from build123d import *

# Parameters (mm, degrees)
SKETCH_W        = 95
SKETCH_H        = 900
PAD_DEPTH       = 45
SKETCH001_W     = 95
SKETCH001_H     = 95
SKETCH001_W_2   = 22.5
SKETCH001_H_2   = 47.5
POCKET_DEPTH    = 22.5
SKETCH011_W     = 22.5
SKETCH011_H     = 47.5
POCKET006_DEPTH = 22.5


with BuildPart() as part:
    # Sketch → Pad (new body)
    with BuildSketch(Plane.XY):
        with Locations((47.5, 450)):
            Rectangle(SKETCH_W, SKETCH_H)
    extrude(amount=-PAD_DEPTH)

    # Sketch001 (on Face5 of Pad) → Pocket (cut)
    with BuildSketch(Plane.XY):
        with Locations((47.5, 167.5)):
            Rectangle(SKETCH001_W, SKETCH001_H)
        with Locations((47.5, 852.5)):
            Rectangle(SKETCH001_W, SKETCH001_H)
        with Locations((47.5, 333.75)):
            Rectangle(SKETCH001_W_2, SKETCH001_H_2)
    extrude(amount=-POCKET_DEPTH, mode=Mode.SUBTRACT)

    # Sketch011 (on Face4 of Pocket) → Pocket006 (cut)
    with BuildSketch(Plane(origin=(0, 0, -45), x_dir=(1, 0, 0), z_dir=(0, 0, -1))):
        with Locations((47.5, -333.75)):
            Rectangle(SKETCH011_W, SKETCH011_H)
    extrude(amount=-POCKET006_DEPTH, mode=Mode.SUBTRACT)


solid = part.part
Input: part model. Units: mm. Frame: model coordinates. A direction names the side the tool comes from. Round coordinates to 2 decimals unless told otherwise and drop trailing zeros. Order: outer loops, then holes, each group sorted by start corner. A loop starts at its lowest first (then second) coordinate and runs counter-clockwise, first axis right, second up. Notation, with made-up numbers: (22, 88) - (30, 88) arc R6 cw to (30, 94) - close; hole circle Ø5 at (-23, 1). An arc over 180 degrees is marked (long way). Answer as a JSON object with one key per item and string values. Group by question number.
(1) Cut plane D-D (y = 130.5). Return loops of the section in (x, z), then the cut area to 3 significant figures.
(2) Reachability of faces 1 (the face through (47, 310, -22)), 2 (the face through (47, 853, -22.5)), 3 (the face through (47, 215, -11)), 4 (the face through (47, 61, 0)) from +Z, -Z, +X, -X, +Y, -Y: full face, straight path, thin tool, end or side. Return the list, or none.
(3) Draft query along Y for faces 5 (the face through (47, 120, -11)), 6 (the face through (47, 805, -11)), 7 (the face through (47, 456, -45)). Return one class per face: released by +Y, released by -Y, zero draft, split by the parting line, or undercut.
(4) Cut plane A-A (z = -14). Return loops of the section in (x, y).
(5) Material intervals for probe 1 along Y at (x, z) = (76, -19.5); probe 2 along Y at (x, z) = (47, -18); probe 3 along Y at (x, z) = (42.5, -42.5), sorted ascending. Write a range as from..to.
(6) Cut plane B-B (x = 72). Return loops of the section in (y, z), then the cut area to 3 significant figures.
(7) Cut plane C-C (y = 318.5). Return loops of the section in (x, z).
(8) Pin query (flat end, axial travel): P1, Ø18, axis at x = 50, z = -12, coming from the +Y side. Return the tip coordinate at first contact, or that it passes through.
Here are the results:
{
 "1": {"outline": "(0, -45) - (95, -45) - (95, -22.5) - (0, -22.5) - close", "area": "2,140 mm^2"},
 "2": {"face 1": "+Z, -Z", "face 2": "+Z, +X, -X, +Y", "face 3": "+Z, +X, -X", "face 4": "+Z, +X, -X, +Y, -Y"},
 "3": {"face 5": "undercut", "face 6": "released by +Y", "face 7": "zero draft"},
 "4": {"outline": "(0, 0) - (95, 0) - (95, 120) - (0, 120) - close; (0, 215) - (95, 215) - (95, 805) - (0, 805) - close; hole (36.25, 310) - (58.75, 310) - (58.75, 357.5) - (36.25, 357.5) - close"},
 "5": {"probe 1": "y = 0..120, 215..805", "probe 2": "y = 0..120, 215..310, 357.5..805", "probe 3": "y = 0..310, 357.5..900"},
 "6": {"outline": "(0, -45) - (900, -45) - (900, -22.5) - (805, -22.5) - (805, 0) - (215, 0) - (215, -22.5) - (120, -22.5) - (120, 0) - (0, 0) - close", "area": "36,200 mm^2"},
 "7": {"outline": "(0, -45) - (36.25, -45) - (36.25, 0) - (0, 0) - close; (58.75, -45) - (95, -45) - (95, 0) - (58.75, 0) - close"},
 "8": {"P1": "stops at y = 805"}
}
